The model under review builds one solid part; all positions refer to its coordinate system, in mm. A direction names the side the tool comes from. Coordinates: 2 decimals unless noted, no trailing zeros. Order: outer loops, then holes, each group sorted by start corner. A loop starts at its lowest first (then second) coordinate and runs counter-clockwise, first axis right, second up. Notation, with made-up numbers: M -11.5,32 L 34.5,32 A23 ccw 34.5,52 Z; hole C 6,33 d5. An arc over 180 degrees is marked long. Write each question's results on one line, items separated by ' | '.
from build123d import *

# Parameters (mm, degrees)
BOSS_EXTRUDE1_DEPTH                          = 10
FILLET1_R                                    = 10
SHELL1_T                                     = -3
FILLET4_R                                    = 3
BOSS_EXTRUDE2_START                          = -3
BOSS_EXTRUDE2_DEPTH                          = 10
BOSS_EXTRUDE6_START                          = -3
BOSS_EXTRUDE6_DEPTH                          = 10
SHELL11_START                                = 3
SHELL11_DEPTH                                = 7
BOSS_EXTRUDE5_DEPTH                          = 3.3
BOSS_EXTRUDE8_DEPTH                          = 3.3
CBORE_FOR_M5_HEX_HEAD_CAP_SCREW4_D           = 3.4
CBORE_FOR_M5_HEX_HEAD_CAP_SCREW4_CBORE_D     = 6.5
CBORE_FOR_M5_HEX_HEAD_CAP_SCREW4_CBORE_DEPTH = 3
SKETCH17_R                                   = 5
BOSS_EXTRUDE4_DEPTH                          = 10
CBORE_FOR_M5_HEX_HEAD_CAP_SCREW3_D           = 3.4
CBORE_FOR_M5_HEX_HEAD_CAP_SCREW3_CBORE_D     = 6.5
CBORE_FOR_M5_HEX_HEAD_CAP_SCREW3_CBORE_DEPTH = 3
CBORE_FOR_M5_HEX_HEAD_CAP_SCREW5_D           = 3.4
CBORE_FOR_M5_HEX_HEAD_CAP_SCREW5_DEPTH       = 5.5
CBORE_FOR_M5_HEX_HEAD_CAP_SCREW5_CBORE_D     = 6.5
CBORE_FOR_M5_HEX_HEAD_CAP_SCREW5_CBORE_DEPTH = 3
CBORE_FOR_M5_HEX_HEAD_CAP_SCREW5_TIP         = 1.021463052


# Read off the part's stored shape, not the designer's step: Shell11
with BuildPart() as part:
    # Sketch1 → Boss-Extrude1 (new body)
    with BuildSketch(Plane.XY):
        with BuildLine():
            Line((17.67766953, -17.67766953), (98.994949366, 63.639610307))
            Line((98.994949366, 63.639610307), (98.994949366, 153.051453663))
            ThreePointArc((98.994949366, 153.051453663), (73.994949366, 178.051453663), (48.994949366, 153.051453663))
            Line((48.994949366, 153.051453663), (48.994949366, 84.350288425))
            Line((48.994949366, 84.350288425), (-17.67766953, 17.67766953))
            ThreePointArc((-17.67766953, 17.67766953), (-17.67766953, -17.67766953), (17.67766953, -17.67766953))
        make_face()
    extrude(amount=BOSS_EXTRUDE1_DEPTH)

    # Fillet1
    fillet1_edges = [part.edges().sort_by_distance(p)[0] for p in [
        (48.994949366, 84.350288425, 5),
        (98.994949366, 63.639610307, 5),
    ]]
    fillet(fillet1_edges, radius=FILLET1_R)

    # Shell1
    shell1_openings = [part.faces().sort_by_distance(p)[0] for p in [
        (50.162308395, 71.072674162, 10),
    ]]
    offset(amount=SHELL1_T, openings=shell1_openings, kind=Kind.INTERSECTION)

    # Fillet4
    fillet4_edges = [part.edges().sort_by_distance(p)[0] for p in [
        (98.994949366, 110.416599797, 0),
        (14.194173824, 49.549512883, 0),
        (98.233744691, 63.954911607, 0),
        (48.233744691, 84.665589726, 0),
        (48.994949366, 120.771938856, 0),
        (73.994949366, 178.051453663, 0),
        (56.871843354, 21.516504294, 0),
        (-17.67766953, -17.67766953, 0),
    ]]
    fillet(fillet4_edges, radius=FILLET4_R)

    # Sketch2 → Boss-Extrude2 (add)
    with BuildSketch(Plane.XY.offset(3).offset(BOSS_EXTRUDE2_START)):
        with BuildLine():
            Line((13.374950088, 22.385502231), (-6.223175758, 9.372010643))
            ThreePointArc((-6.223175758, 9.372010643), (-7.954951288, -7.954951288), (9.372010643, -6.223175758))
            Line((9.372010643, -6.223175758), (22.385502231, 13.374950088))
            ThreePointArc((22.385502231, 13.374950088), (21.566756826, 21.566756826), (13.374950088, 22.385502231))
        make_face()
    extrude(amount=BOSS_EXTRUDE2_DEPTH)

    # Sketch21 → Boss-Extrude6 (add)
    with BuildSketch(Plane.XY.offset(3).offset(BOSS_EXTRUDE6_START)):
        with BuildLine():
            Line((80.366371888, 127.764995329), (85.022411424, 150.824891163))
            ThreePointArc((85.022411424, 150.824891163), (73.994949366, 164.301453663), (62.967487308, 150.824891163))
            Line((62.967487308, 150.824891163), (67.623526844, 127.764995329))
            ThreePointArc((67.623526844, 127.764995329), (73.994949366, 122.551453663), (80.366371888, 127.764995329))
        make_face()
    extrude(amount=BOSS_EXTRUDE6_DEPTH)

    # Shell11 outline → Shell11 (cut)
    with BuildSketch(Plane.XY.offset(SHELL11_START)):
        with BuildLine():
            ThreePointArc((70.564183393, 128.35874533), (73.994949366, 125.551453663), (77.42571534, 128.358745329))
            Line((77.42571534, 128.358745329), (82.081754875, 151.418641163))
            ThreePointArc((82.081754875, 151.418641163), (73.994949366, 161.301453663), (65.908143857, 151.418641163))
            Line((65.908143857, 151.418641163), (70.564183393, 128.35874533))
        make_face()
        with BuildLine():
            Line((15.034463624, 19.886299393), (-4.563662222, 6.872807805))
            ThreePointArc((-4.563662222, 6.872807805), (-5.833630945, -5.833630945), (6.872807805, -4.563662222))
            Line((6.872807805, -4.563662222), (19.886299393, 15.034463624))
            ThreePointArc((19.886299393, 15.034463624), (19.445436483, 19.445436483), (15.034463624, 19.886299393))
        make_face()
    extrude(amount=SHELL11_DEPTH, mode=Mode.SUBTRACT)

    # Sketch18 → Boss-Extrude5 (add)
    with BuildSketch(Plane.XY):
        with BuildLine():
            Line((13.308815704, 22.317827505), (-6.21525525, 9.377265176))
            ThreePointArc((-6.21525525, 9.377265176), (-7.954951288, -7.954951288), (9.377265176, -6.21525525))
            Line((9.377265176, -6.21525525), (22.317827505, 13.308815704))
            ThreePointArc((22.317827505, 13.308815704), (21.496046148, 21.496046148), (13.308815704, 22.317827505))
        make_face()
    extrude(amount=BOSS_EXTRUDE5_DEPTH)

    # Sketch25 → Boss-Extrude8 (add)
    with BuildSketch(Plane.XY):
        with BuildLine():
            Line((80.365282703, 127.859612659), (85.020526295, 150.815575002))
            ThreePointArc((85.020526295, 150.815575002), (73.994949366, 164.301453663), (62.969372437, 150.815575002))
            Line((62.969372437, 150.815575002), (67.624616029, 127.859612659))
            ThreePointArc((67.624616029, 127.859612659), (73.994949366, 122.651453663), (80.365282703, 127.859612659))
        make_face()
    extrude(amount=BOSS_EXTRUDE8_DEPTH)

    # CBORE for M5 Hex Head Cap Screw4 (through all)
    with Locations(Plane(origin=(0, 0, 0), x_dir=(-1, 0, 0), z_dir=(0, 0, -1))):
        with Locations((0, 0), (-16.89985207, 16.89985207)):
            CounterBoreHole(CBORE_FOR_M5_HEX_HEAD_CAP_SCREW4_D / 2, CBORE_FOR_M5_HEX_HEAD_CAP_SCREW4_CBORE_D / 2, CBORE_FOR_M5_HEX_HEAD_CAP_SCREW4_CBORE_DEPTH)

    # Sketch17 → Boss-Extrude4 (add)
    with BuildSketch(Plane.XY):
        with Locations((40.533008589, 58.210678119)):
            Circle(SKETCH17_R)
        with Locations((61.494949366, 108.817279836)):
            Circle(SKETCH17_R)
        with Locations((86.494949366, 108.817279836)):
            Circle(SKETCH17_R)
        with Locations((58.210678119, 40.533008589)):
            Circle(SKETCH17_R)
    extrude(amount=BOSS_EXTRUDE4_DEPTH)

    # CBORE for M5 Hex Head Cap Screw3 (through all)
    with Locations(Plane(origin=(0, 0, 0), x_dir=(-1, 0, 0), z_dir=(0, 0, -1))):
        with Locations((-86.494949366, 108.817279836), (-61.494949366, 108.817279836), (-58.210678119, 40.533008589), (-40.533008589, 58.210678119)):
            CounterBoreHole(CBORE_FOR_M5_HEX_HEAD_CAP_SCREW3_D / 2, CBORE_FOR_M5_HEX_HEAD_CAP_SCREW3_CBORE_D / 2, CBORE_FOR_M5_HEX_HEAD_CAP_SCREW3_CBORE_DEPTH)

    # CBORE for M5 Hex Head Cap Screw5
    with Locations(Plane(origin=(0, 0, 0), x_dir=(-1, 0, 0), z_dir=(0, 0, -1))):
        with Locations((-73.994949366, 153.051453663), (-73.994949366, 129.051453663)):
            CounterBoreHole(CBORE_FOR_M5_HEX_HEAD_CAP_SCREW5_D / 2, CBORE_FOR_M5_HEX_HEAD_CAP_SCREW5_CBORE_D / 2, CBORE_FOR_M5_HEX_HEAD_CAP_SCREW5_CBORE_DEPTH, depth=CBORE_FOR_M5_HEX_HEAD_CAP_SCREW5_DEPTH)
            with Locations((0, 0, -(CBORE_FOR_M5_HEX_HEAD_CAP_SCREW5_DEPTH + CBORE_FOR_M5_HEX_HEAD_CAP_SCREW5_TIP / 2))):  # 118° drill point
                Cone(0, CBORE_FOR_M5_HEX_HEAD_CAP_SCREW5_D / 2, CBORE_FOR_M5_HEX_HEAD_CAP_SCREW5_TIP, mode=Mode.SUBTRACT)


solid = part.part
1) For pin 1 (4 mm diameter, centred on x = 58.21, y = 40.53, fed in from -Z); pin 2 (2 mm diameter, centred on x = 39, y = 60, fed in from -Z); pin 3 (8.5 mm diameter, centred on x = 73.99, y = 153.05, fed in from +Z), all flat-tipped, find the tip position at first contact; note any pin that passes through.
Solutions:
pin 1: z = 3 | pin 2: z = 0 | pin 3: z = 3.3
2) To check wall thickness, follow line 1 along X through (y, z) = (57, 4); line 2 along X through (y, z) = (154.5, 9); line 3 along X through (y, z) = (109, 2). State the ranges of each line that lie inside material, in increasing order.
Solutions:
line 1: 21.64 to 25.89, 35.68 to 39.34, 41.73 to 45.38, 88.11 to 92.36 | line 2: 49.04 to 52.04, 62.84 to 65.87, 82.12 to 85.15, 95.95 to 98.95 | line 3: 49.17 to 58.25, 64.74 to 83.25, 89.74 to 98.82
3) For faces 1 (the flat face through (39, 57, 3)), 2 (the cylindrical face through (-8.15, -7.755, 6.451)), 3 (the flat face through (98.995, 110, 6)), list the 3-axis set-ups (+Z, -Z, +X, -X, +Y, -Y) from which the entire face can be reached by the end or side of a thin tool; tool diameter is ignored.
Solutions:
face 1: -Z | face 2: +Z | face 3: +Z, -Z, +X, +Y, -Y
4) Take a section at B-B on z = 5.5. Count the separate pieces of the cut face and the enclosed holes in it, plus the area to 3 significant figures.
Solutions:
separate pieces: 7 | enclosed holes: 7 | area: 2,390 mm2
5) The part is to be moulded in two halves that separate along Y. For faces 4 (the flat face through (56.323, 20.968, 6.451)), 5 (the flat face through (14.64, 49.996, 6.451)), 6 (the flat face through (48.995, 121, 6)), 7 (the cylindrical face through (2.579, -1.978, 1.479)), say which applies: pulls with the +Y half, pulls with the -Y half, needs draft (parallel to the pull), parting line crosses it, or undercut.
Solutions:
face 4: pulls with the -Y half | face 5: pulls with the +Y half | face 6: needs draft | face 7: undercut
6) Take a section at A-A on y = 117. State the section outline as (x, z) points, plus the area to 3 significant figures.
Solutions:
outline: M 48.99,3 A3 ccw 51.99,0 L 95.99,0 A3 ccw 98.99,3 L 98.99,10 L 95.99,10 L 95.99,3 L 51.99,3 L 51.99,10 L 48.99,10 Z | area: 188 mm2
